Autodesk Inventor part; units mm, degrees
ref_plane "YZ Plane" through (0, 0, 0) normal (1, 0, 0) x (0, 1, 0)
ref_plane "XZ Plane" through (0, 0, 0) normal (0, 1, 0) x (-1, 0, 0)
ref_plane "XY Plane" through (0, 0, 0) normal (0, 0, 1) x (1, 0, 0)
sketch "スケッチ1" plane through (0, 0, 0) normal (0, 1, 0) x (-1, 0, 0)
  line L0 (0, 0) -> (-90, 0)
  line L1 (-90, 0) -> (-90, 50)
  line L2 (0, 50) -> (0, 0)
  line L3 (0, 0) -> (-5, 0)
  line L4 (-5, 0) -> (-5, 50)
  line L5 (-5, 0) -> (-90, 0)
  line L6 (-90, 0) -> (-85, 0)
  line L7 (-85, 0) -> (-85, 50)
  arc A0 (-85, 50) -> (-5, 50) centre (-45, 50) ccw
  line L8 (0, 0) -> (0, 10)
  line L9 (0, 10) -> (-90, 10)
  circle A1 centre (-45, 50) radius 45
  line L10 (-90, 5) -> (0, 5)
  line L11 (-90, 50) -> (-85, 50)
  line L12 (-5, 50) -> (0, 50)
  line L13 (0, 0) -> (-90, 0)
  line L14 (-90, 0) -> (-90, 5)
  line L15 (-90, 5) -> (0, 5)
  line L16 (0, 5) -> (0, 0)
  dimension "d0" = 90
  dimension "d1" = 50
  dimension "d2" = 5
  dimension "d3" = 85
  dimension "d4" = 5
  dimension "d5" = 80
  dimension "d6" = 10
  dimension "d7" = 90
extrude "押し出し1" add sketch "スケッチ1" along normal blind 230 contours L0 L4 L10 L2 | L0 L7 L10 L4 | L10 L4 L9 L2 | L0 L1 L10 L7 | L10 A1 L9 L4 | L9 L4 A1 L2 | L10 L1 L9 L7 | L7 L9 A1 L10 | L9 A1 L4 | A1 L9 | A1 L4 L12 | L9 L1 A1 L7 | L7 A1 L9 | A1 L9 A0 L4 | A1 L7 A0 L9 | L11 L7 A1
sketch "スケッチ2" plane through (0, 0, 0) normal (0, -1, 0) x (1, 0, 0)
  line L0 (0, 0) -> (0, 50)
  line L1 (90, 0) -> (0, 0)
  line L2 (90, 50) -> (90, 0)
  line L3 (85, 50) -> (90, 50)
  arc A0 (5, 50) -> (85, 50) centre (45, 50) ccw
  line L4 (0, 50) -> (5, 50)
  arc A1 (5, 23.467) -> (85, 23.467) centre (45, 50) ccw
  line L5 (0, 5) -> (90, 5)
  line L6 (5, 23.467) -> (5, 5)
  line L7 (85, 23.467) -> (85, 5)
  dimension "d29" = 48
extrude "押し出し2" cut sketch "スケッチ2" against normal blind 225 contours L6 A1 L5 | L5 A1 L7
sketch "スケッチ3" plane through (0, 230, 0) normal (0, 1, 0) x (1, 0, 0)
  arc A0 (85, -50) -> (5, -50) centre (45, -50) ccw
  line L0 (90, -50) -> (90, 0)
  line L1 (0, -50) -> (5, -50)
  arc A1 (85, -50) -> (5, -50) centre (45, -50) ccw
  line L2 (5, -50) -> (85, -50)
extrude "押し出し3" add sketch "スケッチ3" against normal blind 5
sketch "スケッチ4" plane through (90, 0, 50) normal (1, 0, 0) x (0, 0, -1)
  line L0 (0, 0) -> (50, 0)
  line L1 (0, 0) -> (0, 230)
  line L2 (25, 0) -> (25, 65)
  line L3 (25, 65) -> (25, 75)
  line L4 (25, 75) -> (25, 215)
  line L5 (25, 215) -> (25, 225)
  line L6 (0, 65) -> (40, 65)
  line L7 (40, 65) -> (40, 75)
  line L8 (40, 75) -> (0, 75)
  line L9 (0, 75) -> (0, 65)
  line L10 (0, 215) -> (40, 215)
  line L11 (40, 215) -> (40, 225)
  line L12 (40, 225) -> (0, 225)
  line L13 (0, 225) -> (0, 215)
  dimension "d16" = 65
  dimension "d17" = 10
  dimension "d18" = 140
  dimension "d19" = 10
  dimension "d20" = 40
extrude "押し出し4" cut sketch "スケッチ4" against normal blind 90 contours L1 L8 L3 L6 | L3 L8 L7 L6 | L1 L12 L5 L10 | L5 L12 L11 L10
sketch "スケッチ6" plane through (90, 0, 50) normal (1, 0, 0) x (0, 0, -1)
  line L0 (0, 230) -> (50, 230)
  line L1 (50, 230) -> (37.5, 251.6506)
  line L2 (50, 230) -> (110, 230) construction
  line L3 (0, 230) -> (37.5, 251.6506)
  line L4 (0, 230) -> (43.3013, 230) construction
  dimension "d32" = 120
  dimension "d33" = 30
extrude "押し出し6" add sketch "スケッチ6" against normal blind 90
sketch "スケッチ9" plane through (0, 0, 0) normal (-1, 0, 0) x (0, 0, 1)
  line L0 (10, 225) -> (50, 225)
  line L1 (50, 225) -> (50, 230)
  line L2 (50, 230) -> (12.5, 251.6506)
  line L3 (12.5, 251.6506) -> (0, 230)
  line L4 (0, 0) -> (0, 230)
  line L5 (0, 0) -> (50, 0)
  line L6 (50, 0) -> (50, 65)
  line L7 (50, 65) -> (10, 65)
  line L8 (10, 65) -> (10, 75)
  line L9 (10, 75) -> (50, 75)
  line L10 (50, 75) -> (50, 215)
  line L11 (50, 215) -> (10, 215)
  line L12 (10, 215) -> (10, 225)
  line L13 (12.5, 251.6506) -> (0, 230)
  line L14 (0, 230) -> (-132.7906, 0)
  line L15 (0, 145) -> (-49.0748, 145)
  line L16 (0, 115) -> (-66.3953, 115)
  dimension "d45" = 30
sketch "スケッチ10" plane through (0, 0, 0) normal (-1, 0, 0) x (0, 0, 1)
  line L0 (10, 225) -> (50, 225)
  line L1 (50, 225) -> (50, 230)
  line L2 (50, 230) -> (12.5, 251.6506)
  line L3 (12.5, 251.6506) -> (0, 230)
  line L4 (0, 0) -> (0, 230)
  line L5 (0, 0) -> (50, 0)
  line L6 (50, 0) -> (50, 65)
  line L7 (50, 65) -> (10, 65)
  line L8 (10, 65) -> (10, 75)
  line L9 (10, 75) -> (50, 75)
  line L10 (50, 75) -> (50, 215)
  line L11 (50, 215) -> (10, 215)
  line L12 (10, 215) -> (10, 225)
  line L13 (12.5, 251.6506) -> (-87.5, 78.4456)
  line L14 (-87.5, 78.4456) -> (50, 0)
sketch "スケッチ12" plane through (90, 0, 50) normal (1, 0, 0) x (0, 0, -1)
  line L0 (50, 0) -> (50, 230)
  line L1 (40, 225) -> (40, 215)
  line L2 (0, 215) -> (0, 75)
  line L3 (0, 145) -> (50, 145)
  line L4 (32.5, 175) -> (17.5, 175)
  line L5 (17.5, 175) -> (17.5, 115)
  line L6 (17.5, 115) -> (32.5, 115)
  line L7 (32.5, 115) -> (32.5, 175)
  line L8 (32.5, 175) -> (17.5, 115) construction
  line L9 (17.5, 175) -> (32.5, 115) construction
  line L10 (17.5, 145) -> (32.5, 145)
  line L11 (32.5, 145) -> (32.5, 115)
  line L12 (32.5, 115) -> (17.5, 115)
  line L13 (17.5, 115) -> (17.5, 145)
  point P0 (25, 145)
  dimension "d59" = 15
  dimension "d60" = 60
extrude "押し出し8" cut sketch "スケッチ12" against normal blind 2.5 contours L3 L7 L6 L5
sketch "スケッチ13" plane through (0, 0, 0) normal (-1, 0, 0) x (0, 0, 1)
  line L0 (0, 0) -> (0, 230)
  line L1 (50, 75) -> (50, 215)
  line L2 (50, 145) -> (0, 145)
  line L3 (17.5, 175) -> (32.5, 175)
  line L4 (32.5, 175) -> (32.5, 115)
  line L5 (32.5, 115) -> (17.5, 115)
  line L6 (17.5, 115) -> (17.5, 175)
  line L7 (17.5, 175) -> (32.5, 115) construction
  line L8 (32.5, 175) -> (17.5, 115) construction
  line L9 (17.5, 145) -> (32.5, 145)
  line L10 (32.5, 145) -> (32.5, 115)
  line L11 (32.5, 115) -> (17.5, 115)
  line L12 (17.5, 115) -> (17.5, 145)
  point P0 (25, 145)
  dimension "d63" = 15
  dimension "d64" = 60
extrude "押し出し9" cut sketch "スケッチ13" against normal blind 2.5 contours L4 L5 L6 L2
sketch "スケッチ14" plane through (90, 0, 0) normal (0, 0, -1) x (-1, 0, 0)
  line L0 (90, 0) -> (90, 230)
  line L1 (0, 0) -> (0, 230)
  line L2 (0, 145) -> (90, 145)
  line L3 (37.5, 170) -> (52.5, 170)
  line L4 (52.5, 170) -> (52.5, 120)
  line L5 (52.5, 120) -> (37.5, 120)
  line L6 (37.5, 120) -> (37.5, 170)
  line L7 (37.5, 170) -> (52.5, 120) construction
  line L8 (52.5, 170) -> (37.5, 120) construction
  line L9 (37.5, 145) -> (52.5, 145)
  line L10 (52.5, 145) -> (52.5, 170)
  line L11 (52.5, 170) -> (37.5, 170)
  line L12 (37.5, 170) -> (37.5, 145)
  point P0 (45, 145)
  dimension "d67" = 15
  dimension "d70" = 25
extrude "押し出し10" cut sketch "スケッチ14" against normal blind 5 contours L6 L3 L4 L2
sketch "スケッチ16" plane through (90, 0, 0) normal (0, 0, -1) x (-1, 0, 0)
  line L0 (52.5, 170) -> (52.5, 145)
  line L1 (52.5, 145) -> (37.5, 145)
  line L2 (37.5, 145) -> (37.5, 170)
  line L3 (90, 0) -> (90, 230)
  line L4 (0, 0) -> (0, 230)
  line L5 (0, 145) -> (90, 145)
  line L6 (0, 160) -> (37.5, 157.5)
  line L7 (52.5, 157.5) -> (90, 157.5)
  line L8 (18.75, 158.75) -> (18.75, 145)
  line L9 (71.25, 145) -> (71.25, 157.5)
  line L10 (11.25, 175) -> (26.25, 175)
  line L11 (26.25, 175) -> (26.25, 115)
  line L12 (26.25, 115) -> (11.25, 115)
  line L13 (11.25, 115) -> (11.25, 175)
  line L14 (11.25, 175) -> (26.25, 115) construction
  line L15 (26.25, 175) -> (11.25, 115) construction
  line L16 (11.25, 115) -> (26.25, 115)
  line L17 (26.25, 115) -> (26.25, 175)
  line L18 (26.25, 175) -> (11.25, 175)
  line L19 (11.25, 175) -> (11.25, 115)
  line L20 (45, 145) -> (45, 125)
  line L21 (78.75, 175) -> (63.75, 175)
  line L22 (63.75, 115) -> (78.75, 115)
  line L23 (78.75, 175) -> (78.75, 115)
  line L24 (63.75, 115) -> (63.75, 175)
  line L25 (63.75, 175) -> (78.75, 175)
  line L26 (78.75, 175) -> (78.75, 115)
  line L27 (78.75, 115) -> (63.75, 115)
  line L28 (63.75, 115) -> (63.75, 175)
  line L29 (11.25, 115) -> (26.25, 115)
  line L30 (26.25, 115) -> (26.25, 175)
  line L31 (26.25, 175) -> (11.25, 175)
  line L32 (11.25, 175) -> (11.25, 115)
  dimension "d71" = 15
  dimension "d72" = 60
  dimension "d73" = 20
extrude "押し出し11" cut sketch "スケッチ16" against normal blind 3 contours L24 L21 L23 L7 | L7 L9 L5 L24 | L5 L23 L22 L24 | L7 L23 L5 L9 | L11 L12 L13 L5 | L5 L8 L6 L11 | L6 L13 L10 L11 | L5 L13 L6 L8
sketch "スケッチ17" plane through (37.5, 145, 0) normal (0, 1, 0) x (1, 0, 0)
  line L0 (-57.7643, 16.522) -> (69.053, 16.522)
  line L1 (69.053, 16.522) -> (69.053, -65.9751)
  line L2 (69.053, -65.9751) -> (-57.7643, -65.9751)
  line L3 (-57.7643, -65.9751) -> (-57.7643, 16.522)
  point P0 (-37.5, 0)
extrude "押し出し12" cut sketch "スケッチ17" against normal blind 180
sketch "スケッチ18" plane through (0, 215, 10) normal (-1, 0, 0) x (0, 0, 1)
  line L0 (-10, -70) -> (40, -70)
  line L1 (7.5, -40) -> (22.5, -40)
  line L2 (22.5, -40) -> (22.5, -100)
  line L3 (22.5, -100) -> (7.5, -100)
  line L4 (7.5, -100) -> (7.5, -40)
  line L5 (7.5, -40) -> (22.5, -100) construction
  line L6 (22.5, -40) -> (7.5, -100) construction
  point P0 (-10, -215)
  point P1 (15, -70)
  dimension "d78" = 15
  dimension "d79" = 60
extrude "押し出し13" add sketch "スケッチ18" against normal blind 2.5
sketch "スケッチ19" plane through (90, 215, 10) normal (1, 0, 0) x (0, 0, -1)
  line L0 (-40, -70) -> (10, -70)
  line L1 (-22.5, -40) -> (-7.5, -40)
  line L2 (-7.5, -40) -> (-7.5, -100)
  line L3 (-7.5, -100) -> (-22.5, -100)
  line L4 (-22.5, -100) -> (-22.5, -40)
  line L5 (-22.5, -40) -> (-7.5, -100) construction
  line L6 (-7.5, -40) -> (-22.5, -100) construction
  point P0 (10, -215)
  point P1 (-15, -70)
  dimension "d82" = 15
  dimension "d83" = 60
extrude "押し出し14" add sketch "スケッチ19" against normal blind 2.5
sketch "スケッチ20" plane through (90, 230, 0) normal (0, 0.5, -0.8660254) x (-1, 0, 0)
  line L0 (0, 0) -> (0, 25)
  line L1 (0, 0) -> (90, 0)
  line L2 (90, 25) -> (90, 0)
  line L3 (0, 25) -> (90, 25)
  line L4 (0, 12.5) -> (90, 12.5)
  line L5 (45, 12.5) -> (45, 25)
  line L6 (45, 12.5) -> (45, 0)
  line L7 (22.5, 18.5) -> (67.5, 18.5)
  line L8 (67.5, 18.5) -> (67.5, 6.5)
  line L9 (67.5, 6.5) -> (22.5, 6.5)
  line L10 (22.5, 6.5) -> (22.5, 18.5)
  line L11 (22.5, 18.5) -> (67.5, 6.5) construction
  line L12 (67.5, 18.5) -> (22.5, 6.5) construction
  circle A0 centre (45, 6.5) radius 3
  circle A1 centre (67.5, 18.5) radius 3
  circle A2 centre (67.5, 6.5) radius 3
  circle A3 centre (22.5, 6.5) radius 3
  circle A4 centre (22.5, 18.5) radius 3
  circle A5 centre (45, 18.5) radius 3
  point P0 (90, -199.1858)
  dimension "d86" = 45
  dimension "d87" = 6
  dimension "d89" = 6
  dimension "d90" = 6
  dimension "d91" = 6
  dimension "d92" = 6
  dimension "d93" = 6
  dimension "d94" = 6
extrude "押し出し15" add sketch "スケッチ20" along normal blind 4 contours A0 L9 L6 | L6 L9 A0 | A3 L9 L10 | L10 L9 A3 | A4 L7 L10 | L10 L7 A4 | L9 A0 L6 | L6 A0 L9 | A5 L7 L5 | L5 L7 A5 | A5 L7 L5 | L5 L7 A5 | A2 L8 L9 | L9 L8 A2 | A1 L7 L8 | L8 L7 A1
ref_plane "作業平面2" through (45, 160, 50) normal (0, -1, 0) x (1, 0, 0)
sketch "スケッチ21" plane through (45, 160, 50) normal (0, -1, 0) x (1, 0, 0)
  line L0 (-52.9668, 19.8142) -> (54.3752, 19.8142)
  line L1 (54.3752, 19.8142) -> (54.3752, -61.5309)
  line L2 (54.3752, -61.5309) -> (-52.9668, -61.5309)
  line L3 (-52.9668, -61.5309) -> (-52.9668, 19.8142)
  line L4 (-52.9668, 19.8142) -> (54.3752, -61.5309) construction
  line L5 (54.3752, 19.8142) -> (-52.9668, -61.5309) construction
  point P0 (-45, -50)
  point P1 (0.7042, -20.8583)
extrude "押し出し16" cut sketch "スケッチ21" along normal blind 50
sketch "スケッチ22" plane through (90, 215, 10) normal (1, 0, 0) x (0, 0, -1)
  line L0 (-40, -55) -> (10, -55)
  line L1 (-22.5, -25) -> (-7.5, -25)
  line L2 (-7.5, -25) -> (-7.5, -85)
  line L3 (-7.5, -85) -> (-22.5, -85)
  line L4 (-22.5, -85) -> (-22.5, -25)
  line L5 (-22.5, -25) -> (-7.5, -85) construction
  line L6 (-7.5, -25) -> (-22.5, -85) construction
  point P0 (10, -215)
  point P1 (-15, -55)
  dimension "d100" = 15
  dimension "d101" = 60
extrude "押し出し17" cut sketch "スケッチ22" against normal blind 2.5
sketch "スケッチ23" plane through (0, 215, 10) normal (-1, 0, 0) x (0, 0, 1)
  line L0 (-10, -55) -> (40, -55)
  line L1 (7.5, -25) -> (22.5, -25)
  line L2 (22.5, -25) -> (22.5, -85)
  line L3 (22.5, -85) -> (7.5, -85)
  line L4 (7.5, -85) -> (7.5, -25)
  line L5 (7.5, -25) -> (22.5, -85) construction
  line L6 (22.5, -25) -> (7.5, -85) construction
  point P0 (-10, -215)
  point P1 (15, -55)
  dimension "d104" = 15
  dimension "d105" = 60
extrude "押し出し18" cut sketch "スケッチ23" against normal blind 2.5
properties part number "知能ロボコン発射台２.11" material "ABS プラスチック"
For this review, take the finished solid that the model builds, in its own axes (mm). A direction names the side the tool comes from. Round coordinates to 2 decimals unless told otherwise and drop trailing zeros. Order: outer loops, then holes, each group sorted by start corner. A loop starts at its lowest first (then second) coordinate and runs counter-clockwise, first axis right, second up. Notation, with made-up numbers: M 2.5,35.25 L 43.5,35.25 A24 cw 43.5,49.25 Z; hole C 89,-15.5 d7. An arc over 180 degrees is marked long. Write each question's results on one line, items separated by ' | '. Start each with the question number.
1. Add section D-D (y = 217). State the section outline as (x, z) points.
2. Add section C-C (z = 37.5). State the section outline as (x, y) points.
3. Tool access review of faces 4 (the face through (78.75, 167, 1)), 5 (the face through (88, 220, 10)), 6 (the face through (89, 175, 17.5)), 7 (the face through (2.5, 175, 25)), 8 (the face through (44, 195, 0)): name each direction out of +Z, -Z, +X, -X, +Y, -Y from which nothing blocks a thin tool from reaching the whole face with its end or side.
4. To check wall thickness, follow L1, parallel to X at y = 208.5, z = 21; L2, parallel to X at y = 222.5, z = 7; L3, parallel to X at y = 190.5, z = 19. State the ranges of each line that lie inside material, in increasing order. Write a range as [from, to].
5. Add section A-A (x = 73). State the section outline as (y, z) points.
6. Draft analysis for pull direction Y (two halves, no side actions). For faces 1 (the face through (19.73, 237.61, 2.12)), 2 (the face through (16, 192, 5)), 3 (the face through (45, 170, 2)), state which applies: pulls with the +Y half, pulls with the -Y half, needs draft (parallel to the pull), parting line crosses it, or undercut.
7. Add section B-B (y = 199.5). State the section outline as (x, z) points.
8. Clearance check with flat-ended pins moving along their axes: pin 1 Ø8 at (x, z) = (52, 39) entering from -Y; pin 2 Ø5 at (x, y) = (68.5, 237.5) entering from +Z; pin 3 Ø8 at (x, y) = (72.5, 200) entering from +Z. State where each tip first meets the part, or that it passes through.
Output values:
1) outline: M 0,0 L 90,0 L 90,10 L 85,10 L 85,5 L 61.7,5 A48 ccw 71.53,10 L 18.47,10 A48 ccw 28.3,5 L 5,5 L 5,10 L 0,10 Z
2) outline: M 0,160 L 7,160 L 7,215 L 0,215 Z; M 0,225 L 90,225 L 90,237.22 L 0,237.22 Z; M 83,160 L 90,160 L 90,215 L 83,215 Z
3) face 4: -Z, -Y | face 5: +Z, +X, -X | face 6: +X, -Y | face 7: -X, -Y | face 8: -Z, +X, -X, -Y
4) L1: [0, 5], [6.75, 17.45], [72.55, 83.25], [85, 90] | L2: [0, 5], [23.67, 66.33], [85, 90] | L3: [0, 5], [8.35, 19.72], [70.28, 81.65], [85, 90]
5) outline: M 160,3 L 175,3 L 175,0 L 230,0 L 251.65,12.5 L 230,50 L 225,50 L 225,5 L 160,5 Z; M 160,11.01 L 215,11.01 L 215,21.43 L 160,21.43 Z
6) face 1: undercut | face 2: needs draft | face 3: pulls with the -Y half
7) outline: M 0,0 L 90,0 L 90,50 L 85,50 A40 cw 5,50 L 0,50 Z; hole M 5,5 L 28.3,5 A48 cw 5,23.47 Z; hole M 61.7,5 L 85,5 L 85,23.47 A48 cw Z
8) pin 1: y = 225 | pin 2: z = 41.34 | pin 3: z = 25.35
